from build123d import *

# Parameters (mm, degrees)
SKETCH_1_W             = 8
SKETCH_1_H             = 8
HEIGHT_DEPTH           = 3.2
SKETCH_2_R             = 2.4
EXTRUDE_2_DEPTH        = 1.7
PATTERN_LINEAR_1_COUNT = 4
PATTERN_LINEAR_1_PITCH = 8
SHELL_1_T              = -1.6


with BuildPart() as part:
    # 草圖1 → height (new body)
    with BuildSketch(Plane(origin=(0, 0, 0), x_dir=(1, 0, 0), z_dir=(0, 1, 0))):
        Rectangle(SKETCH_1_W, SKETCH_1_H)
    height = extrude(amount=HEIGHT_DEPTH)

    # 草圖2 → 填料-伸長2 (add)
    with BuildSketch(Plane(origin=(0, 3.2, 0), x_dir=(1, 0, 0), z_dir=(0, 1, 0))):
        Circle(SKETCH_2_R)
    extrude_2 = extrude(amount=EXTRUDE_2_DEPTH)

    # 直線複製排列1: height, 填料-伸長2 ×4
    with Locations(*[(i * PATTERN_LINEAR_1_PITCH, 0, 0) for i in range(1, PATTERN_LINEAR_1_COUNT)]):
        add(height)
        add(extrude_2)

    # 薄殼1
    shell_1_openings = [part.faces().sort_by_distance(p)[0] for p in [
        (12, 0, 0),
    ]]
    offset(amount=SHELL_1_T, openings=shell_1_openings, kind=Kind.INTERSECTION)


solid = part.part
The listing builds one solid part. Answer for the finished solid, in the listing's coordinates (mm). A direction names the side the tool comes from. Give positions to 0.01 mm unless a question says otherwise; leave off trailing zeros. Order: outer loops, then holes, each group sorted by start corner. A loop starts at its lowest first (then second) coordinate and runs counter-clockwise, first axis right, second up. Notation, with made-up numbers: (-20, 84.25) - (21, 84.25) arc R24 cw to (21, 96.25) - close; hole circle Ø10 at (-0.75, 1.5). An arc over 180 degrees is marked (long way). Answer as CSV lines item,"result".
Q1. Which of the six approach directions +Z, -Z, +X, -X, +Y, -Y give full straight-line access (tool end or side, diameter ignored) to faces 4 (the face through (15.2, 2.4, 0)), 5 (the face through (12, 0, -3)), 6 (the face through (12, 3.2, 0))?
Answer key:
face 4,"-Y"
face 5,"+Z, -Z, +X, -X, -Y"
face 6,"+Y"
Q2. A cutting plane is placed at B-B, the plane x = 21. Determine the outline of the cut face in (y, z).
Answer key:
outline,"(0, -4) - (3.2, -4) - (3.2, 4) - (0, 4) - (0, 2.4) - (1.6, 2.4) - (1.6, -2.4) - (0, -2.4) - close"
Q3. Straight lines are drawn through the part: L1, parallel to X at y = 4.3, z = -0.5; L2, parallel to X at y = 4.3, z = 0; L3, parallel to Z at x = 16, y = 2.75. For each, find the intervals that lie inside material, in ascending order.
Answer key:
L1,"x = -2.35 to 2.35, 5.65 to 10.35, 13.65 to 18.35, 21.65 to 26.35"
L2,"x = -2.4 to 2.4, 5.6 to 10.4, 13.6 to 18.4, 21.6 to 26.4"
L3,"z = -4 to -0.8, 0.8 to 4"
Q4. Each of these flat-tipped pins is pushed along its axis until it touches: pin 1 Ø2 at (x, z) = (3.5, -2) entering from +Y; pin 2 Ø0.8 at (x, z) = (0, 0) entering from -Y; pin 3 Ø1.3 at (x, z) = (24, -0.5) entering from -Y. Where does it stop, or does it pass through?
Answer key:
pin 1,"stops at y = 3.2"
pin 2,"stops at y = 3.3"
pin 3,"stops at y = 1.6"
Q5. A cutting plane is placed at C-C, the plane z = 2. Determine the outline of the cut face in (x, y).
Answer key:
outline,"(-4, 0) - (-2.4, 0) - (-2.4, 1.6) - (26.4, 1.6) - (26.4, 0) - (28, 0) - (28, 3.2) - (25.33, 3.2) - (25.33, 4.9) - (22.67, 4.9) - (22.67, 3.2) - (17.33, 3.2) - (17.33, 4.9) - (14.67, 4.9) - (14.67, 3.2) - (9.33, 3.2) - (9.33, 4.9) - (6.67, 4.9) - (6.67, 3.2) - (1.33, 3.2) - (1.33, 4.9) - (-1.33, 4.9) - (-1.33, 3.2) - (-4, 3.2) - close"
Q6. A cutting plane is placed at A-A, the plane y = 0.9. Determine the outline of the cut face in (x, z), and give its area (3 significant figures).
Answer key:
outline,"(-4, -4) - (28, -4) - (28, 4) - (-4, 4) - close; hole (-2.4, -2.4) - (26.4, -2.4) - (26.4, 2.4) - (-2.4, 2.4) - close"
area,"118 mm^2"
Q7. Determine the mould class of faces 1 (the face through (12, 1, 2.4)), 2 (the face through (0, 4.9, 0)), 3 (the face through (13.602, 4.038, -0.106)) for opening direction Z: pulls with the +Z half, pulls with the -Z half, needs draft (parallel to the pull), parting line crosses it, or undercut.
Answer key:
face 1,"undercut"
face 2,"needs draft"
face 3,"parting line crosses it"
Q8. A cutting plane is placed at D-D, the plane x = 8. Determine the outline of the cut face in (y, z).
Answer key:
outline,"(0, -4) - (3.2, -4) - (3.2, -2.4) - (4.9, -2.4) - (4.9, 2.4) - (3.2, 2.4) - (3.2, 4) - (0, 4) - (0, 2.4) - (1.6, 2.4) - (1.6, 0.8) - (3.3, 0.8) - (3.3, -0.8) - (1.6, -0.8) - (1.6, -2.4) - (0, -2.4) - close"
